```python
from build123d import *

# Parameters (mm, degrees)
RESSALTO_EXTRUS_O1_DEPTH = 3
CORTE_EXTRUS_O2_DEPTH    = 151.026697624
ESBO_O5_R                = 1.5
CORTE_EXTRUS_O3_DEPTH    = 93.556406403


with BuildPart() as part:
    # Esboço1 → Ressalto-extrusão1 (new body)
    with BuildSketch(Plane(origin=(0, 0, 0), x_dir=(1, 0, 0), z_dir=(0, 1, 0))):
        Polygon((-75, 0), (75, 0), (0, 129.9), align=None)
    extrude(amount=RESSALTO_EXTRUS_O1_DEPTH)

    # Esboço4 → Corte-extrusão2 (cut, through all)
    with BuildSketch(Plane(origin=(0, 3, 0), x_dir=(1, 0, 0), z_dir=(0, 1, 0))):
        Polygon((-28.742601802, 80.117813679), (28.742601802, 80.117813679), (0, 129.9), align=None)
        Polygon((-46.239258354, 49.813604531), (-17.548607665, 0), (-75, 0), align=None)
        Polygon((17.532230415, 0), (75, 0), (46.247424766, 49.799460305), align=None)
    extrude(amount=-CORTE_EXTRUS_O2_DEPTH, mode=Mode.SUBTRACT)

    # Esboço5 → Corte-extrusão3 (cut, through all)
    with BuildSketch(Plane(origin=(0, 3, 0), x_dir=(1, 0, 0), z_dir=(0, 1, 0))):
        with Locations(Location((-26.806110129, 76.617813679, 0), (0, 0, 270))):
            Circle(ESBO_O5_R)
        with Locations(Location((26.806110129, 76.617813679, 0), (0, 0, 90))):
            Circle(ESBO_O5_R)
        with Locations(Location((-15.612115992, 3.5, 0), (0, 0, 270))):
            Circle(ESBO_O5_R)
        with Locations(Location((15.612115992, 3.5, 0), (0, 0, 90))):
            Circle(ESBO_O5_R)
    extrude(amount=-CORTE_EXTRUS_O3_DEPTH, mode=Mode.SUBTRACT)


solid = part.part
```
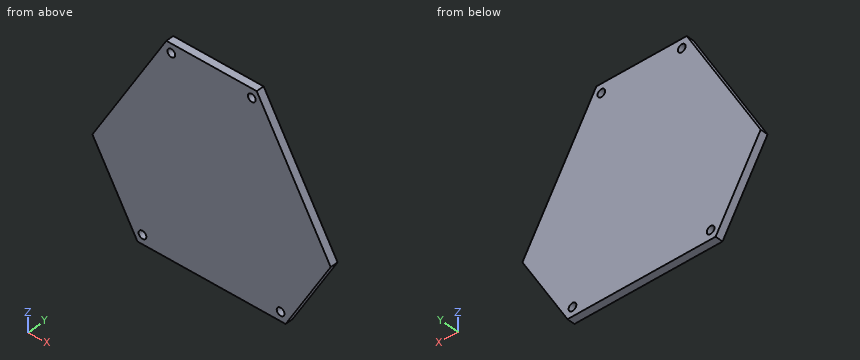
Read the model definition and answer for the solid it produces. Units are mm, in the model's axes. Give positions to 0.01 mm unless a question says otherwise; leave off trailing zeros. Write each loop counter-clockwise with the first axis right and the second up, starting at its lowest first coordinate (ties: lowest second). Pieces come first, ordered by that corner, then holes. Notation, with made-up numbers: M 50.25,0.25 L 87.25,0.25 A18 ccw 87.25,17.25 Z; hole C 16.25,80.25 d3. An arc over 180 degrees is marked long. Put each result on its own line as item: value. Start each with the question number.
1. Each of these flat-tipped pins is pushed along its axis until it touches: pin 1 Ø3 at (x, z) = (-29, -17) entering from +Y; pin 2 Ø1 at (y, z) = (2, -10.5) entering from +X (3 decimals). Where does it stop, or does it pass through?
2. The part is cut by section A-A, the plane z = -3.5. Give the vertices of the cut face in (x, y), and give its area (3 significant figures).
3. The part is cut by section B-B, the plane y = 1.4. Give the vertices of the cut face in (x, z).
4. Consider line 1 along X through (y, z) = (1.1, -3.5); line 2 along Z through (x, y) = (15.5, 0.8); line 3 along Z through (x, y) = (-16.5, 0.7). Determine where each line is inside the solid, lowest interval first.
5. The part is cut by section C-C, the plane z = -20. Give the vertices of the cut face in (x, y).
Final values:
1. pin 1: stops at y = 3
1. pin 2: stops at x = 23.875
2. outline: M -19.56,0 L -17.11,0 L -17.11,3 L -19.56,3 Z; M -14.11,0 L 14.11,0 L 14.11,3 L -14.11,3 Z; M 17.11,0 L 19.55,0 L 19.55,3 L 17.11,3 Z
2. area: 99.3 mm²
3. outline: M -46.24,-49.81 L -28.74,-80.12 L 28.74,-80.12 L 46.25,-49.8 L 17.53,0 L -17.55,0 Z; hole C -26.81,-76.62 d3; hole C -15.61,-3.5 d3; hole C 15.61,-3.5 d3; hole C 26.81,-76.62 d3
4. line 1: x = -19.56 to -17.11, -14.11 to 14.11, 17.11 to 19.55
4. line 2: z = -80.12 to -5, -2 to 0
4. line 3: z = -80.12 to -4.71, -2.29 to 0
5. outline: M -29.07,0 L 29.06,0 L 29.06,3 L -29.07,3 Z
